```python
from build123d import *

# Parameters (mm, degrees)
SKETCH_1_R      = 1.6
EXTRUDE_1_DEPTH = 3
FILLET_1_R      = 2
FILLET_2_R      = 5


with BuildPart() as part:
    # 草图1 → 凸台-拉伸1 (new body)
    with BuildSketch(Plane(origin=(0, 0, 0), x_dir=(1, 0, 0), z_dir=(0, 1, 0))):
        Polygon((0, -50), (-20, -50), (-20, 40), (50, 40), (50, 0), align=None)
        with Locations(Location((-10, -5, 0), (0, 0, 270))):
            Circle(SKETCH_1_R, mode=Mode.SUBTRACT)
        with Locations(Location((-10, -25, 0), (0, 0, 270))):
            Circle(SKETCH_1_R, mode=Mode.SUBTRACT)
        with Locations(Location((-10, -45, 0), (0, 0, 270))):
            Circle(SKETCH_1_R, mode=Mode.SUBTRACT)
        with Locations(Location((-10, 10, 0), (0, 0, 270))):
            Circle(SKETCH_1_R, mode=Mode.SUBTRACT)
        with Locations(Location((-10, 30, 0), (0, 0, 270))):
            Circle(SKETCH_1_R, mode=Mode.SUBTRACT)
        with Locations(Location((10, 30, 0), (0, 0, 270))):
            Circle(SKETCH_1_R, mode=Mode.SUBTRACT)
        with Locations(Location((10, 10, 0), (0, 0, 270))):
            Circle(SKETCH_1_R, mode=Mode.SUBTRACT)
        with Locations(Location((30, 30, 0), (0, 0, 270))):
            Circle(SKETCH_1_R, mode=Mode.SUBTRACT)
        with Locations(Location((30, 10, 0), (0, 0, 270))):
            Circle(SKETCH_1_R, mode=Mode.SUBTRACT)
        Polygon((0, -38.686291501), (0, 0), (38.686291501, 0), align=None, mode=Mode.SUBTRACT)
    extrude(amount=EXTRUDE_1_DEPTH)

    # 圆角1
    fillet_1_edges = [part.edges().sort_by_distance(p)[0] for p in [
        (0, 1.5, 50),
        (-20, 1.5, 50),
        (-20, 1.5, -40),
        (50, 1.5, -40),
        (50, 1.5, 0),
    ]]
    fillet(fillet_1_edges, radius=FILLET_1_R)

    # 圆角2
    fillet_2_edges = [part.edges().sort_by_distance(p)[0] for p in [
        (38.686291501, 1.5, 0),
        (0, 1.5, 0),
        (0, 1.5, 38.686291501),
    ]]
    fillet(fillet_2_edges, radius=FILLET_2_R)


solid = part.part
```
For this review, take the finished solid that the model builds, in its own axes (mm). A direction names the side the tool comes from. Round coordinates to 2 decimals unless told otherwise and drop trailing zeros. Write each loop counter-clockwise with the first axis right and the second up, starting at its lowest first coordinate (ties: lowest second). Pieces come first, ordered by that corner, then holes.
1) For line 1 along X through (y, z) = (1.45, -10); line 2 along X through (y, z) = (1.1, 45); line 3 along Z through (x, y) = (-11, 2.05), list the stretches that pass through material, from the lowest coordinate up.
Answer below:
line 1: x = -20 to -11.6, -8.4 to 8.4, 11.6 to 28.4, 31.6 to 50
line 2: x = -20 to -11.6, -8.4 to 5
line 3: z = -40 to -31.25, -28.75 to -11.25, -8.75 to 3.75, 6.25 to 23.75, 26.25 to 43.75, 46.25 to 50
2) Mouldability with a two-part tool opening along Z and no side actions: class faces 1 (the face through (-10.97, 1.48, -11.27)), 2 (the face through (49.43, 1.52, -39.4)), 3 (the face through (25, 1, 25)), 4 (the face through (-20, 1, 6)) as +Z half, -Z half, draft (parallel to the pull), parting line (faces both ways), or undercut.
Answer below:
face 1: undercut
face 2: -Z half
face 3: +Z half
face 4: draft
3) Take a section at B-B on x = -10. Give the boundary of the cut face in (y, z), then the cut area to 3 significant figures.
Answer below:
outline: (0, -40) - (3, -40) - (3, -31.6) - (0, -31.6) - close; (0, -28.4) - (3, -28.4) - (3, -11.6) - (0, -11.6) - close; (0, -8.4) - (3, -8.4) - (3, 3.4) - (0, 3.4) - close; (0, 6.6) - (3, 6.6) - (3, 23.4) - (0, 23.4) - close; (0, 26.6) - (3, 26.6) - (3, 43.4) - (0, 43.4) - close; (0, 46.6) - (3, 46.6) - (3, 50) - (0, 50) - close
area: 222 mm2
4) Take a section at D-D on y = 0.85. State how many separate pieces and enclosed holes the cut face has, then the cut area to 3 significant figures.
Answer below:
separate pieces: 1
enclosed holes: 10
area: 4,290 mm2
5) Machinability: for faces 5 (the face through (19.494, 1.479, 19.192)), 6 (the face through (8, 0, -6)), which of the approach directions +Z, -Z, +X, -X, +Y, -Y give a long, thin tool a straight path to every point of the face, cutting with its end or side? Answer none if there is none.
Answer below:
face 5: +Y, -Y
face 6: +Z, -Z, +X, -X, -Y
6) Insertion check: pin 1 Ø12 at (x, z) = (6, 31.5) entering from -Y; pin 2 Ø1.5 at (x, y) = (16, 1.5) entering from +Z. Each pin has a flat end and moves straight along its axis. Give the tip position at first contact, or say it passes through.
Answer below:
pin 1: stops at y = 0
pin 2: stops at z = 34.75
7) Take a section at C-C on z = 45. Give the boundary of the cut face in (x, y), then the cut area to 3 significant figures.
Answer below:
outline: (-20, 0) - (-11.6, 0) - (-11.6, 3) - (-20, 3) - close; (-8.4, 0) - (5, 0) - (5, 3) - (-8.4, 3) - close
area: 65.4 mm2
8) Take a section at A-A on z = -10. Give the boundary of the cut face in (x, y), then the cut area to 3 significant figures.
Answer below:
outline: (-20, 0) - (-11.6, 0) - (-11.6, 3) - (-20, 3) - close; (-8.4, 0) - (8.4, 0) - (8.4, 3) - (-8.4, 3) - close; (11.6, 0) - (28.4, 0) - (28.4, 3) - (11.6, 3) - close; (31.6, 0) - (50, 0) - (50, 3) - (31.6, 3) - close
area: 181 mm2
